Design review of the part built by this model. Coordinates are the model's own, in mm. Give positions to 0.01 mm unless a question says otherwise; leave off trailing zeros. Put each result on its own line as item: value. Start each with the question number.
from build123d import *

# Parameters (mm, degrees)
F0_W     = 90
F0_H     = 90
F1_DEPTH = 1300
F2_R     = 5.25
F3_DEPTH = 1
F4_R     = 10.25
F5_DEPTH = 90.001


with BuildPart() as f1:
    # F0 (on Top) → F1 (new body)
    with BuildSketch(Plane.XY):
        Rectangle(F0_W, F0_H)
    extrude(amount=F1_DEPTH)

    # F2 (on face) → F3 (cut)
    with BuildSketch(Plane.XZ.offset(45)):
        with Locations((0, 1225)):
            Circle(F2_R)
        with Locations((0, 175)):
            Circle(F2_R)
    extrude(amount=-F3_DEPTH, mode=Mode.SUBTRACT)

    # F4 (on face) → F5 (cut, through all)
    with BuildSketch(Plane(origin=(-45, 0, 0), x_dir=(0, -1, 0), z_dir=(-1, 0, 0))):
        with Locations((0, 100)):
            Circle(F4_R)
        with Locations((0, 200)):
            Circle(F4_R)
    extrude(amount=-F5_DEPTH, mode=Mode.SUBTRACT)


solid = f1.part
1. To check wall thickness, follow probe 1 along Z at (x, y) = (0, -44.45); probe 2 along Z at (x, y) = (-19, 0). State the ranges of each line that lie inside material, in increasing order.
2. The part is to be moulded in two halves that separate along Z. For faces 1 (the flat face through (45, -1, 641)), 2 (the cylindrical face through (-0.63, 1.334, 110.163)), 3 (the flat face through (-1, 1, 0)), say which applies: +Z half, -Z half, draft (parallel to the pull), parting line (faces both ways), or undercut.
3. Insertion check: pin 1 (23.5 mm diameter, centred on y = 0, z = 100, fed in from -X); pin 2 (16.5 mm diameter, centred on y = 0, z = 200, fed in from +X); pin 3 (5 mm diameter, centred on x = 0, z = 172.5, fed in from -Y). Each pin has a flat end and moves straight along its axis. Give the tip position at first contact, or say it passes through.
Returned:
1. probe 1: z = 0 to 169.75, 180.25 to 1219.75, 1230.25 to 1300
1. probe 2: z = 0 to 89.75, 110.25 to 189.75, 210.25 to 1300
2. face 1: draft
2. face 2: undercut
2. face 3: -Z half
3. pin 1: stops at x = -45
3. pin 2: passes through
3. pin 3: stops at y = -44
